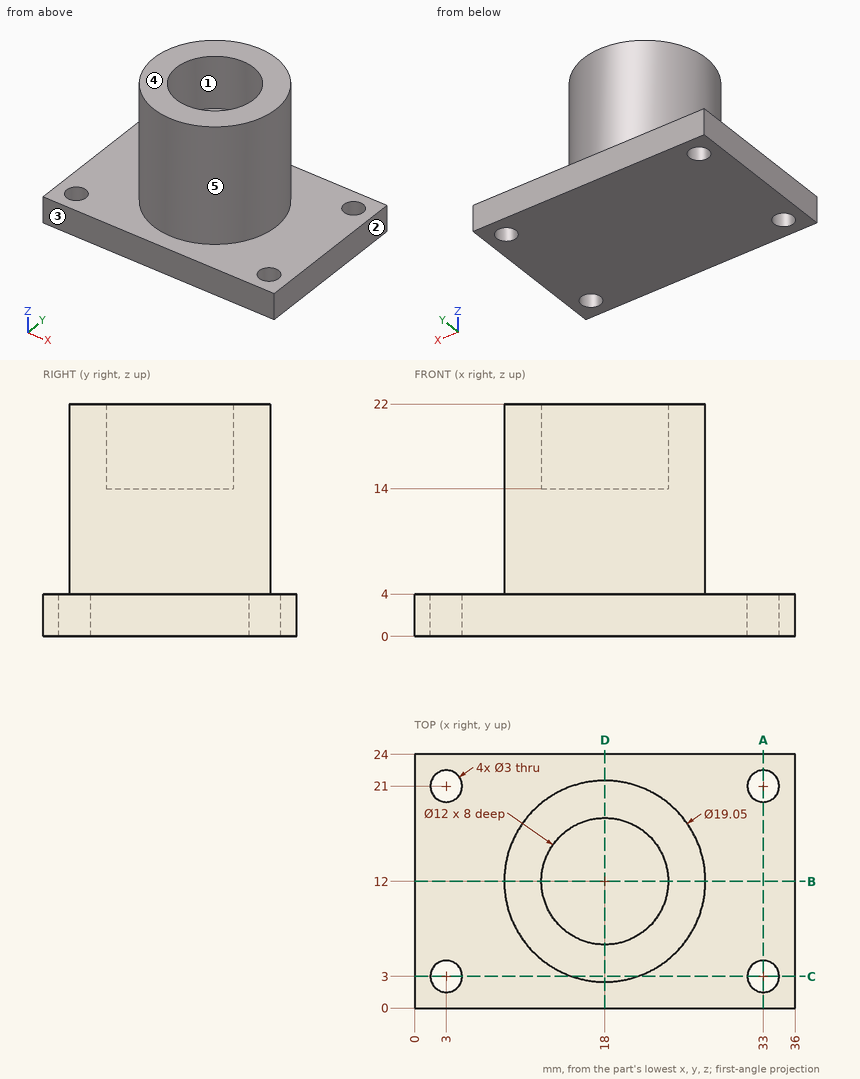
Can you work these out from the drawing? Everything is in mm from the part's minimum corner. A direction names the side the tool comes from. Coordinates: 2 decimals unless noted, no trailing zeros. Loops run counter-clockwise (first coordinate to the right, second up) from the corner with the lowest first, then second, coordinate; pieces in that order, holes last. Notation, with made-up numbers: (6, 86.25) - (50, 86.25) arc R11 ccw to (50, 96.25) - close; hole circle Ø2 at (10.25, -2.75). An arc over 180 degrees is marked (long way). Answer as CSV lines item,"result".
Q1. If I drill on L1, parallel to X at y = 21, z = 3.05; L2, parallel to Y at x = 33, z = 2.25; L3, parallel to Z at x = 10.5, y = 4.75, over which ranges is the centre line in solid material (lowest first)? Write a range as [from, to].
Response:
L1,"[0, 1.5], [4.5, 31.5], [34.5, 36]"
L2,"[0, 1.5], [4.5, 19.5], [22.5, 24]"
L3,"[0, 4]"
Q2. If we section it at C-C, the plane y = 3: Write out the boundary of the cut face in (x, z), and give its area (3 significant figures).
Response:
outline,"(0, 0) - (1.5, 0) - (1.5, 4) - (0, 4) - close; (4.5, 0) - (31.5, 0) - (31.5, 4) - (21.12, 4) - (21.12, 22) - (14.88, 22) - (14.88, 4) - (4.5, 4) - close; (34.5, 0) - (36, 0) - (36, 4) - (34.5, 4) - close"
area,"232 mm2"
Q3. If we section it at B-B, the plane y = 12: Write out the boundary of the cut face in (x, z) (3 decimals), and give its area (3 significant figures).
Response:
outline,"(0, 0) - (36, 0) - (36, 4) - (27.525, 4) - (27.525, 22) - (24, 22) - (24, 14) - (12, 14) - (12, 22) - (8.475, 22) - (8.475, 4) - (0, 4) - close"
area,"391 mm2"
Q4. For the marked faces 4 and 5, which set-ups out of +Z, -Z, +X, -X, +Y, -Y let a thin tool reach every point of the face, with its end or its side?
Response:
face 4,"+Z, +X, -X, +Y, -Y"
face 5,"+Z"
Q5. If we section it at D-D, the plane x = 18: Write out the boundary of the cut face in (y, z) (3 decimals).
Response:
outline,"(0, 0) - (24, 0) - (24, 4) - (21.525, 4) - (21.525, 22) - (18, 22) - (18, 14) - (6, 14) - (6, 22) - (2.475, 22) - (2.475, 4) - (0, 4) - close"
Q6. For pin 1 (3 mm diameter, centred on y = 12, z = 7, fed in from -X) (3 decimals); pin 2 (1 mm diameter, centred on y = 3.5, z = 11, fed in from +X); pin 3 (1.5 mm diameter, centred on x = 17.5, y = 21.5, fed in from -Z); pin 4 (2.5 mm diameter, centred on x = 3, y = 3, fed in from -Z), each with a flat end and sliding along its axis, tell me the tip position at first contact or that it passes through.
Response:
pin 1,"x = 8.475"
pin 2,"x = 23.17"
pin 3,"z = 0"
pin 4,"through"
Q7. If we section it at A-A, the plane x = 33: Write out the boundary of the cut face in (y, z).
Response:
outline,"(0, 0) - (1.5, 0) - (1.5, 4) - (0, 4) - close; (4.5, 0) - (19.5, 0) - (19.5, 4) - (4.5, 4) - close; (22.5, 0) - (24, 0) - (24, 4) - (22.5, 4) - close"
Q8. We'd pull the mould along Y, two halves only. Please class the marked faces 1, 2 and 3: pulls with the +Y half, pulls with the -Y half, needs draft (parallel to the pull), parting line crosses it, or undercut.
Response:
face 1,"undercut"
face 2,"needs draft"
face 3,"pulls with the -Y half"
